Autodesk Inventor part; units mm, degrees
ref_plane "YZ Plane" through (0, 0, 0) normal (1, 0, 0) x (0, 1, 0)
ref_plane "XZ Plane" through (0, 0, 0) normal (0, 1, 0) x (-1, 0, 0)
ref_plane "XY Plane" through (0, 0, 0) normal (0, 0, 1) x (1, 0, 0)
sketch "Sketch1" plane through (0, 0, 0) normal (0, 1, 0) x (-1, 0, 0)
  line L0 (59.2667, 296.3333) -> (-42.3333, 296.3333)
  line L1 (-42.3333, 296.3333) -> (-42.3333, -84.6667)
  line L2 (-42.3333, -84.6667) -> (59.2667, -84.6667)
  line L3 (59.2667, -84.6667) -> (59.2667, 296.3333)
  point P0 (0, 0)
  dimension "d0" = 101.6
  dimension "d1" = 381
extrude "Plate1" add sketch "Sketch1" along normal blind 6.35
sketch "Sketch2" plane through (35.9833, 0, -84.6667) normal (1, 0, 0) x (0, 1, 0)
  line L0 (0, 381) -> (0, 0)
  line L1 (0, 0) -> (101.6, 0)
  line L2 (101.6, 0) -> (101.6, 381)
  line L3 (101.6, 381) -> (0, 381)
edge flange "Flange1" height 101.6 angle 90 thickness 6.35 bend radius 0.0254 thickness toward (1, 0, 0) relief straight relief width 6.35 relief depth 3.175 edges at (42.3333, 6.35, 105.8333) wall of the first edge with corners at (35.9833, 0, 296.3333) (35.9833, 0, -84.6667) (35.9833, 101.6, -84.6667) (35.9833, 101.6, 296.3333)
bend "Bend1"
corner "Corner1"
sketch "Sketch3" plane through (42.3333, 101.6, 296.3333) normal (1, 0, 0) x (0, 0, -1)
  line L0 (20.0406, 0) -> (378.4346, 0) construction
  line L1 (378.4346, 0) -> (378.4346, -101.6) construction
  line L2 (378.4346, -101.6) -> (20.0406, -101.6) construction
  line L3 (20.0406, -101.6) -> (20.0406, 0) construction
  line L4 (0, -95.2246) -> (0, 0) construction
  line L5 (0, 0) -> (381, 0) construction
  line L6 (20.0406, 0) -> (83.5406, 0) construction
  line L7 (83.5406, 0) -> (83.5406, -95.25) construction
  line L8 (83.5406, -95.25) -> (20.0406, -95.25) construction
  line L9 (20.0406, -95.25) -> (20.0406, 0) construction
  line L10 (118.3386, 0) -> (181.8386, 0) construction
  line L11 (181.8386, 0) -> (181.8386, -95.25) construction
  line L12 (181.8386, -95.25) -> (118.3386, -95.25) construction
  line L13 (118.3386, -95.25) -> (118.3386, 0) construction
  line L14 (216.6366, 0) -> (280.1366, 0) construction
  line L15 (280.1366, 0) -> (280.1366, -95.25) construction
  line L16 (280.1366, -95.25) -> (216.6366, -95.25) construction
  line L17 (216.6366, -95.25) -> (216.6366, 0) construction
  line L18 (314.9346, 0) -> (378.4346, 0) construction
  line L19 (378.4346, 0) -> (378.4346, -95.25) construction
  line L20 (378.4346, -95.25) -> (314.9346, -95.25) construction
  line L21 (314.9346, -95.25) -> (314.9346, 0) construction
  line L22 (35.9156, -25.4) -> (67.6656, -25.4) construction
  line L23 (134.4168, -25.4) -> (166.1668, -25.4) construction
  line L24 (232.918, -25.4) -> (264.668, -25.4) construction
  line L25 (331.4192, -25.4) -> (363.1692, -25.4) construction
  point P0 (296.3333, -101.6)
  dimension "d13" = 358.394
  dimension "d14" = 20.0406
  dimension "d15" = 101.6
  dimension "d16" = 0
  dimension "d17" = 63.5
  dimension "d18" = 63.5
  dimension "d19" = 34.798
  dimension "d20" = 63.5
  dimension "d21" = 34.798
  dimension "d22" = 63.5
  dimension "d23" = 34.798
  dimension "d24" = 25.4
  dimension "d25" = 31.75
  dimension "d26" = 15.875
  dimension "d36" = 98.5012
hole "Hole1" at (42.3333, 76.2, 260.4177) at (42.3333, 76.2, 228.6677) at (42.3333, 76.2, 130.1665) at (42.3333, 76.2, 161.9165) at (42.3333, 76.2, 63.4153) at (42.3333, 76.2, 31.6653) at (42.3333, 76.2, -35.0859) at (42.3333, 76.2, -66.8359) direction (-1, 0, 0) diameter 3.9624 depth 13.6144 tip angle 118
sketch "Sketch4" plane through (0, 6.35, 0) normal (0, 1, 0) x (1, 0, 0)
  line L0 (-59.2667, -296.3333) -> (-59.2667, 84.6667)
  line L1 (-59.2667, 84.6667) -> (35.9579, 84.6667)
  line L2 (42.3333, -296.3333) -> (42.3333, 84.6667)
  line L3 (35.9579, -296.3333) -> (-59.2667, -296.3333)
  point P0 (7.4083, 59.2667)
  point P1 (7.4083, -16.9333)
  point P2 (7.4083, -67.7333)
  point P3 (7.4083, -143.9333)
  point P4 (7.4083, -194.7333)
  point P5 (7.4083, -270.9333)
  dimension "d42" = 25.4
  dimension "d45" = 76.2
  dimension "d58" = 34.925
  dimension "d59" = 34.925
  dimension "d60" = 50.8
  dimension "d61" = 76.2
  dimension "d62" = 50.8
  dimension "d63" = 76.2
  dimension "d64" = 25.4
  dimension "d65" = 34.925
  dimension "d66" = 34.925
  dimension "d67" = 34.925
hole "Hole2" at (7.4083, 6.35, -59.2667) at (7.4083, 6.35, 16.9333) at (7.4083, 6.35, 67.7333) at (7.4083, 6.35, 143.9333) at (7.4083, 6.35, 194.7333) at (7.4083, 6.35, 270.9333) direction (0, -1, 0) diameter 3.9624 depth 13.6144 tip angle 118
equation "\"d3\" = BendReliefWidth"
equation "\"d4\" = BendReliefDepth"
equation "\"d5\" = MinimumRemnant"
equation "\"d6\" = BendRadius"
equation "\"d10\" = CornerReliefSize"
equation "\"d11\" = GapSize"
equation "\"d12\" = JacobiRadiusSize"
equation "\"BendRadius\" = Thickness"
equation "\"BendReliefWidth\" = Thickness"
equation "\"BendReliefDepth\" = 0.5 * Thickness"
equation "\"CornerReliefSize\" = 4 * Thickness"
equation "\"MinimumRemnant\" = 2 * Thickness"
equation "\"TransitionRadius\" = BendRadius"
equation "\"JacobiRadiusSize\" = Thickness"
equation "\"GapSize\" = Thickness"
equation "\"d2\" = BendRadius"
properties part number "ubracket"
Can you work these out from the model? Positions are in its coordinate system, mm. A direction names the side the tool comes from. Round coordinates to 2 decimals unless told otherwise and drop trailing zeros. Loops run counter-clockwise (first coordinate to the right, second up) from the corner with the lowest first, then second, coordinate; pieces in that order, holes last. Notation, with made-up numbers: (88, 78.25) -> (129, 78.25) arc R31 ccw to (129, 115.25) -> close; hole circle Ø11 at (82.5, 1.25). An arc over 180 degrees is marked (long way). One line per item, written item: value. Start each with the question number.
1. For faces 1 (the flat face through (-11, 6.35, 109)), 2 (the flat face through (-11, 0, 109)), which set-ups out of +Z, -Z, +X, -X, +Y, -Y let a thin tool reach every point of the face, with its end or its side?
2. For pin 1 (4.5 mm diameter, centred on x = 7.41, z = 67.73, fed in from +Y); pin 2 (3.5 mm diameter, centred on y = 76.2, z = 130.17, fed in from -X); pin 3 (5 mm diameter, centred on y = 83.5, z = 162.5, fed in from -X), each with a flat end and sliding along its axis, tell me the tip position at first contact or that it passes through.
3. If I drill on probe 1 along Y at (x, z) = (15, 160); probe 2 along X at (y, z) = (49, 70); probe 3 along X at (y, z) = (4, 191), over which ranges is the centre line in solid material (lowest first)?
4. If we section it at C-C, the plane y = 94: Write out the boundary of the cut face in (x, z), then the cut area to 3 significant figures.
5. If we section it at B-B, the plane x = -23: Write out the boundary of the cut face in (y, z), then the cut area to 3 significant figures.
Calculated:
1. face 1: +Z, -Z, -X, +Y
1. face 2: +Z, -Z, +X, -X, -Y
2. pin 1: stops at y = 6.35
2. pin 2: passes through
2. pin 3: stops at x = 35.98
3. probe 1: y = 0 to 6.35
3. probe 2: x = 35.98 to 42.33
3. probe 3: x = -59.27 to 41.87
4. outline: (35.98, -84.67) -> (42.33, -84.67) -> (42.33, 296.33) -> (35.98, 296.33) -> close
4. area: 2,420 mm²
5. outline: (0, -84.67) -> (6.35, -84.67) -> (6.35, 296.33) -> (0, 296.33) -> close
5. area: 2,420 mm²
